Design review of the part built by this model. Coordinates are the model's own, in mm. A direction names the side the tool comes from. Give positions to 0.01 mm unless a question says otherwise; leave off trailing zeros. Order: outer loops, then holes, each group sorted by start corner. A loop starts at its lowest first (then second) coordinate and runs counter-clockwise, first axis right, second up. Notation, with made-up numbers: (55.25, -13) -> (92.25, -13) arc R26 cw to (92.25, 6) -> close; hole circle Ø8 at (88, 11). An arc over 180 degrees is marked (long way). One line per item, written item: value. Start each with the question number.
1) Consider section C-C (z = -2). State the section outline as (x, y) points.
2) Consider section B-B (x = 2.54). State the section outline as (y, z) points, plus the area to 3 significant figures.
3) The part is to be moulded in two halves that separate along X. For faces 1 (the face through (8.747, 5.706, -8.206)), 2 (the face through (10, 3, 0)), 3 (the face through (0, 3, -5)), say which applies: released by +X, released by -X, zero draft, split by the parting line, or undercut.
4) Consider section A-A (z = -7.62). State the section outline as (x, y) points, plus the area to 3 significant figures.
5) Wall thickness on line 1 along X through (y, z) = (5.5, -7); line 2 along Y through (x, z) = (11, -2.25); line 3 along Z through (x, y) = (3, 6.25): over which ranges is each line inside the solid? List them lowest first. Write a range as from..to.
6) Tool access review of faces 4 (the face through (19.02, 5.71, -2.26)), 5 (the face through (3, 6.35, -8)): name each direction out of +Z, -Z, +X, -X, +Y, -Y from which nothing blocks a thin tool from reaching the whole face with its end or side.
7) Consider section D-D (x = 11). State the section outline as (y, z) points, plus the area to 3 significant figures.
from build123d import *

# Parameters (mm, degrees)
SKETCH1_W            = 20.32
SKETCH1_H            = 10.16
BOSS_EXTRUDE1_DEPTH  = 5.08
SKETCH2_R            = 1.27
BOSS_EXTRUDE2_DEPTH  = 1.27
LPATTERN1_COUNT      = 4
LPATTERN1_PITCH      = 5.08
LPATTERN1_COUNT_DIR2 = 2
LPATTERN1_PITCH_DIR2 = 5.08


with BuildPart() as part:
    # Sketch1 → Boss-Extrude1 (new body)
    with BuildSketch(Plane(origin=(0, 0, 0), x_dir=(1, 0, 0), z_dir=(0, 1, 0))):
        with Locations((10.16, 5.08)):
            Rectangle(SKETCH1_W, SKETCH1_H)
    extrude(amount=BOSS_EXTRUDE1_DEPTH)

    # Sketch2 → Boss-Extrude2 (add)
    with BuildSketch(Plane(origin=(0, 5.08, 0), x_dir=(1, 0, 0), z_dir=(0, 1, 0))):
        with Locations(Location((2.54, 2.54, 0), (0, 0, 90))):
            Circle(SKETCH2_R)
    boss_extrude2 = extrude(amount=BOSS_EXTRUDE2_DEPTH)

    # LPattern1: Boss-Extrude2 4 × 2
    with Locations(*[(i * LPATTERN1_PITCH, 0, -j * LPATTERN1_PITCH_DIR2) for i in range(LPATTERN1_COUNT) for j in range(LPATTERN1_COUNT_DIR2) if (i, j) != (0, 0)]):
        add(boss_extrude2)


solid = part.part
Checked values:
1. outline: (0, 0) -> (20.32, 0) -> (20.32, 5.08) -> (18.93, 5.08) -> (18.93, 6.35) -> (16.63, 6.35) -> (16.63, 5.08) -> (13.85, 5.08) -> (13.85, 6.35) -> (11.55, 6.35) -> (11.55, 5.08) -> (8.77, 5.08) -> (8.77, 6.35) -> (6.47, 6.35) -> (6.47, 5.08) -> (3.69, 5.08) -> (3.69, 6.35) -> (1.39, 6.35) -> (1.39, 5.08) -> (0, 5.08) -> close
2. outline: (0, -10.16) -> (5.08, -10.16) -> (5.08, -8.89) -> (6.35, -8.89) -> (6.35, -6.35) -> (5.08, -6.35) -> (5.08, -3.81) -> (6.35, -3.81) -> (6.35, -1.27) -> (5.08, -1.27) -> (5.08, 0) -> (0, 0) -> close
2. area: 58.1 mm^2
3. face 1: undercut
3. face 2: zero draft
3. face 3: released by -X
4. outline: (0, 0) -> (20.32, 0) -> (20.32, 5.08) -> (19.05, 5.08) -> (19.05, 6.35) -> (16.51, 6.35) -> (16.51, 5.08) -> (13.97, 5.08) -> (13.97, 6.35) -> (11.43, 6.35) -> (11.43, 5.08) -> (8.89, 5.08) -> (8.89, 6.35) -> (6.35, 6.35) -> (6.35, 5.08) -> (3.81, 5.08) -> (3.81, 6.35) -> (1.27, 6.35) -> (1.27, 5.08) -> (0, 5.08) -> close
4. area: 116 mm^2
5. line 1: x = 1.43..3.65, 6.51..8.73, 11.59..13.81, 16.67..18.89
5. line 2: y = 0..5.08
5. line 3: z = -8.8..-6.44, -3.72..-1.36
6. face 4: +Y
6. face 5: +Z, -Z, +X, -X, +Y
7. outline: (0, -10.16) -> (5.08, -10.16) -> (5.08, 0) -> (0, 0) -> close
7. area: 51.6 mm^2
